from build123d import *

# Parameters (mm, degrees)
SKETCH1_W           = 45
SKETCH1_H           = 50
BOSS_EXTRUDE1_DEPTH = 45
SKETCH2_R           = 5.2
CUT_EXTRUDE1_DEPTH  = 45
SKETCH9_R           = 5.15
CUT_EXTRUDE6_DEPTH  = 2
SKETCH10_R          = 5.15
CUT_EXTRUDE7_DEPTH  = 2
SKETCH12_R          = 18.375
CUT_EXTRUDE8_DEPTH  = 45
SKETCH13_W          = 45
SKETCH13_H          = 6.66747138
CUT_EXTRUDE9_DEPTH  = 46
SKETCH14_W          = 45
SKETCH14_H          = 6.66747138
BOSS_EXTRUDE2_DEPTH = 45
SKETCH15_R          = 18.375
CUT_EXTRUDE10_DEPTH = 45
FILLET1_R           = 15
SKETCH16_R          = 18.375
BOSS_EXTRUDE3_DEPTH = 2
SKETCH17_R          = 11.5
CUT_EXTRUDE11_DEPTH = 2
SKETCH18_R          = 1.8
CUT_EXTRUDE12_DEPTH = 2


with BuildPart() as part:
    # Sketch1 → Boss-Extrude1 (new body)
    with BuildSketch(Plane.XY):
        with Locations((8.236607143, -2.901785714)):
            Rectangle(SKETCH1_W, SKETCH1_H)
    extrude(amount=BOSS_EXTRUDE1_DEPTH)

    # Sketch2 → Cut-Extrude1 (cut)
    with BuildSketch(Plane.XY.offset(45)):
        with Locations((-4.163392857, -24.901785714)):
            Circle(SKETCH2_R)
        with Locations((20.636607143, -24.901785714)):
            Circle(SKETCH2_R)
    extrude(amount=-CUT_EXTRUDE1_DEPTH, mode=Mode.SUBTRACT)

    # Sketch9 → Cut-Extrude6 (cut)
    with BuildSketch(Plane.XY.offset(45)):
        with Locations((8.236607143, -2.401785714)):
            Circle(SKETCH9_R)
    extrude(amount=-CUT_EXTRUDE6_DEPTH, mode=Mode.SUBTRACT)

    # Sketch10 → Cut-Extrude7 (cut)
    with BuildSketch(Plane(origin=(0, 0, 0), x_dir=(-1, 0, 0), z_dir=(0, 0, -1))):
        with Locations((-8.236607143, -2.401785714)):
            Circle(SKETCH10_R)
    extrude(amount=-CUT_EXTRUDE7_DEPTH, mode=Mode.SUBTRACT)

    # Sketch12 → Cut-Extrude8 (cut)
    with BuildSketch(Plane.ZY.offset(14.263392857)):
        with Locations((22.5, 1.098214286)):
            Circle(SKETCH12_R)
    extrude(amount=-CUT_EXTRUDE8_DEPTH, mode=Mode.SUBTRACT)

    # Sketch13 → Cut-Extrude9 (cut)
    with BuildSketch(Plane.ZY.offset(14.263392857)):
        with Locations((22.5, 18.764478596)):
            Rectangle(SKETCH13_W, SKETCH13_H)
    extrude(amount=-CUT_EXTRUDE9_DEPTH, mode=Mode.SUBTRACT)

    # Sketch14 → Boss-Extrude2 (add)
    with BuildSketch(Plane.ZY.offset(14.263392857)):
        with Locations((22.5, 18.764478596)):
            Rectangle(SKETCH14_W, SKETCH14_H)
    extrude(amount=-BOSS_EXTRUDE2_DEPTH)

    # Sketch15 → Cut-Extrude10 (cut)
    with BuildSketch(Plane.ZY.offset(14.263392857)):
        with Locations((22.5, 1.098214286)):
            Circle(SKETCH15_R)
    extrude(amount=-CUT_EXTRUDE10_DEPTH, mode=Mode.SUBTRACT)

    # Fillet1
    fillet1_edges = [part.edges().sort_by_distance(p)[0] for p in [
        (8.236607143, 22.098214286, 0),
        (8.236607143, 22.098214286, 45),
    ]]
    fillet(fillet1_edges, radius=FILLET1_R)

    # Sketch16 → Boss-Extrude3 (add)
    with BuildSketch(Plane(origin=(30.736607143, 0, 0), x_dir=(0, 0, -1), z_dir=(1, 0, 0))):
        with Locations((-22.5, 1.098214286)):
            Circle(SKETCH16_R)
    extrude(amount=-BOSS_EXTRUDE3_DEPTH)

    # Sketch17 → Cut-Extrude11 (cut)
    with BuildSketch(Plane(origin=(30.736607143, 0, 0), x_dir=(0, 0, -1), z_dir=(1, 0, 0))):
        with Locations((-22.5, 1.098214286)):
            Circle(SKETCH17_R)
    extrude(amount=-CUT_EXTRUDE11_DEPTH, mode=Mode.SUBTRACT)

    # Sketch18 → Cut-Extrude12 (cut)
    with BuildSketch(Plane(origin=(30.736607143, 0, 0), x_dir=(0, 0, -1), z_dir=(1, 0, 0))):
        with Locations((-22.5, 15.098214286)):
            Circle(SKETCH18_R)
    extrude(amount=-CUT_EXTRUDE12_DEPTH, mode=Mode.SUBTRACT)


solid = part.part
The model under review builds one solid part; all positions refer to its coordinate system, in mm. A direction names the side the tool comes from. Round coordinates to 2 decimals unless told otherwise and drop trailing zeros. Loops run counter-clockwise (first coordinate to the right, second up) from the corner with the lowest first, then second, coordinate; pieces in that order, holes last. Notation, with made-up numbers: (40, 61.25) - (66, 61.25) arc R5 cw to (66, 67.25) - close; hole circle Ø7 at (42.5, -32). An arc over 180 degrees is marked (long way). Use CSV: the item, a comma, the result in double quotes.
(1) Clearance check with flat-ended pins moving along their axes: P1, Ø1, axis at x = 16.5, y = 8, coming from the +Z side; P2, Ø1.5, axis at x = -6.5, z = 37, coming from the -Y side. State where each tip first meets the part, or that it passes through.
Working result:
P1,"stops at z = 44.99"
P2,"stops at y = -20.72"
(2) Machinability: for faces 1 (the flat face through (28.737, -11, 23)), 2 (the cylindrical face through (3.324, -0.855, 0.986)), 3 (the cylindrical face through (4.44, 1.08, 44.01)), 4 (the flat face through (8, -11, 0)), 5 (the flat face through (28, -27.902, 22)), which of the approach directions +Z, -Z, +X, -X, +Y, -Y give a long, thin tool a straight path to every point of the face, cutting with its end or side? Answer none if there is none.
Working result:
face 1,"-X"
face 2,"-Z"
face 3,"+Z"
face 4,"-Z, +X, -X, +Y, -Y"
face 5,"+Z, -Z, +X, -X, -Y"
(3) Take a section at A-A, the plane z = 22.5. Give the boundary of the cut face in (x, y), plus the area to 3 significant figures.
Working result:
outline,"(-14.26, -27.9) - (-8.41, -27.9) arc R5.2 cw (long way) to (0.08, -27.9) - (16.39, -27.9) arc R5.2 cw (long way) to (24.88, -27.9) - (30.74, -27.9) - (30.74, -10.4) - (28.74, -10.4) - (28.74, -17.28) - (-14.26, -17.28) - close; (-14.26, 19.47) - (28.74, 19.47) - (28.74, 16.9) - (30.74, 16.9) - (30.74, 22.1) - (-14.26, 22.1) - close; (28.74, 12.6) - (30.74, 12.6) - (30.74, 13.3) - (28.74, 13.3) - close"
area,"473 mm^2"
(4) Take a section at B-B, the plane y = 4. Give the boundary of the cut face in (x, z), plus the area to 3 significant figures.
Working result:
outline,"(-14.26, 0) - (30.74, 0) - (30.74, 11.37) - (28.74, 11.37) - (28.74, 4.36) - (-14.26, 4.36) - close; (-14.26, 40.64) - (28.74, 40.64) - (28.74, 33.63) - (30.74, 33.63) - (30.74, 45) - (-14.26, 45) - close"
area,"420 mm^2"
(5) Take a section at D-D, the plane y = -14. Give the boundary of the cut face in (x, z), plus the area to 3 significant figures.
Working result:
outline,"(-14.26, 0) - (30.74, 0) - (30.74, 45) - (-14.26, 45) - (-14.26, 32.97) - (28.74, 32.97) - (28.74, 12.03) - (-14.26, 12.03) - close"
area,"1,120 mm^2"
(6) Take a section at C-C, the plane x = -2.5. Give the boundary of the cut face in (y, z) (3 decimals).
Working result:
outline,"(-19.975, 0) - (7.098, 0) arc R15 ccw to (22.098, 15) - (22.098, 30) arc R15 ccw to (7.098, 45) - (-19.975, 45) - close; hole circle Ø36.75 at (1.098, 22.5)"
(7) For line 1 (Y direction, x = 30.15, z = 22.5); line 2 (Y direction, x = 30, z = 22); line 3 (Y direction, x = 3, z = 14), list the stretches that pass through material, from the lowest coordinate up.
Working result:
line 1,"y = -27.9 to -10.4, 12.6 to 13.3, 16.9 to 22.1"
line 2,"y = -27.9 to -10.39, 12.59 to 13.37, 16.83 to 22.1"
line 3,"y = -27.9 to -15.19, 17.39 to 22.06"
(8) The part is to be moulded in two halves that separate along Z. For faces 6 (the cylindrical face through (8.55, 17.59, 4.28)), 7 (the cylindrical face through (6.936, 18.223, 29.163)), 8 (the cylindrical face through (8.55, 17.59, 40.72)), say which applies: pulls with the +Z half, pulls with the -Z half, needs draft (parallel to the pull), parting line crosses it, or undercut.
Working result:
face 6,"pulls with the -Z half"
face 7,"undercut"
face 8,"pulls with the +Z half"
